For this review, use the dimensioned drawing (mm, ordinates from the lowest corner) and the shaded views. Give positions to 0.01 mm unless a question says otherwise; leave off trailing zeros. Order: outer loops, then holes, each group sorted by start corner. A loop starts at its lowest first (then second) coordinate and runs counter-clockwise, first axis right, second up. Notation, with made-up numbers: (-22, 0.5) - (21, 0.5) arc R16 ccw to (21, 17.5) - close; hole circle Ø2 at (63, 2). An arc over 180 degrees is marked (long way). Use a Markdown table: item, result. Add a question column.
1) We need section D-D on x = 68. Write out the cut boundary in (y, z).
2) We need section C-C on z = 2.4. Give the number of separate pieces and of enclosed holes in the cut face, then the cut area to 3 significant figures.
3) Wall thickness on L1, parallel to Y at x = 7, z = 2.75; L2, parallel to Y at x = 51, z = 1.6; L3, parallel to Y at x = 73, z = 3.3 (1 decimal): over which ranges is each line inside the solid? List them lowest first.
4) We need section A-A on x = 7. Write out the cut boundary in (y, z).
5) We need section B-B on y = 21. Write out the cut boundary in (x, z), then the cut area to 3 significant figures.
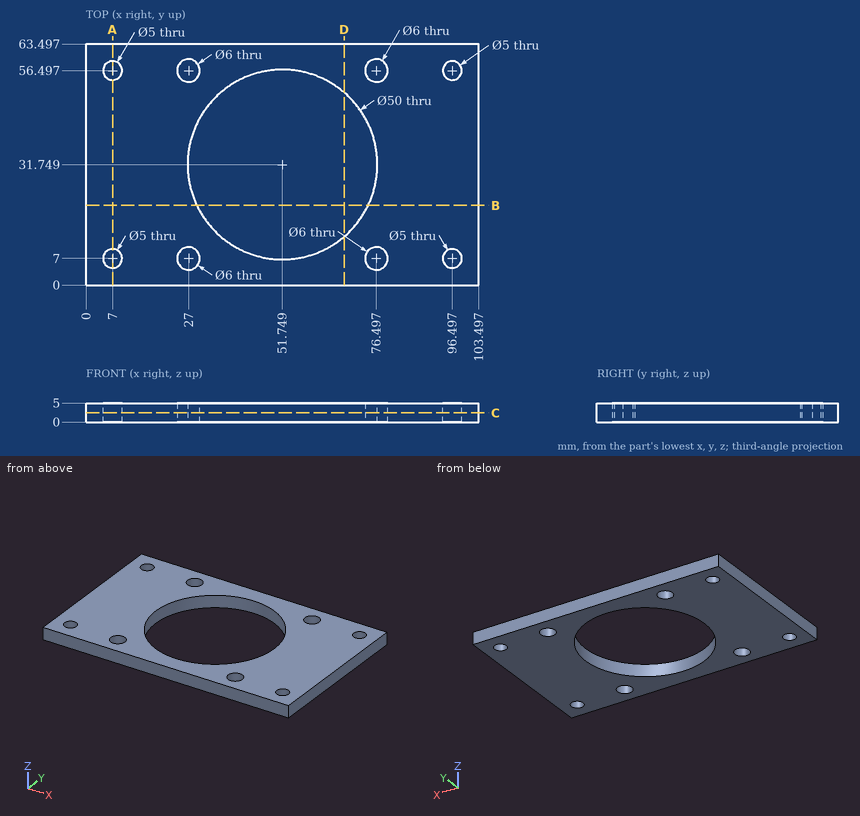
Checked values:
| question | item | result |
|---|---|---|
| 1 | outline | (0, 0) - (12.75, 0) - (12.75, 5) - (0, 5) - close; (50.75, 0) - (63.5, 0) - (63.5, 5) - (50.75, 5) - close |
| 2 | separate pieces | 1 |
| 2 | enclosed holes | 9 |
| 2 | area | 4,420 mm² |
| 3 | L1 | 0 to 4.5, 9.5 to 54, 59 to 63.5 |
| 3 | L2 | 0 to 6.76, 56.74 to 63.5 |
| 3 | L3 | 0 to 18.6, 44.9 to 63.5 |
| 4 | outline | (0, 0) - (4.5, 0) - (4.5, 5) - (0, 5) - close; (9.5, 0) - (54, 0) - (54, 5) - (9.5, 5) - close; (59, 0) - (63.5, 0) - (63.5, 5) - (59, 5) - close |
| 5 | outline | (0, 0) - (29.18, 0) - (29.18, 5) - (0, 5) - close; (74.32, 0) - (103.5, 0) - (103.5, 5) - (74.32, 5) - close |
| 5 | area | 292 mm² |
